Autodesk Inventor part; units mm, degrees
ref_plane "YZ Plane" through (0, 0, 0) normal (1, 0, 0) x (0, 1, 0)
ref_plane "XZ Plane" through (0, 0, 0) normal (0, 1, 0) x (-1, 0, 0)
ref_plane "XY Plane" through (0, 0, 0) normal (0, 0, 1) x (1, 0, 0)
sketch "Boceto1" plane through (0, 0, 0) normal (0, 1, 0) x (-1, 0, 0)
  line L0 (8, 8.175) -> (-8, 8.175)
  line L1 (-8, 8.175) -> (-8, -8.175)
  line L2 (-8, -8.175) -> (8, -8.175)
  line L3 (8, -8.175) -> (8, 8.175)
  point P0 (0, 0)
  dimension "d0" = 16.35
  dimension "d1" = 16
  dimension "d2" = 8
  dimension "d3" = 8.175
extrude "Extrusión1" add sketch "Boceto1" along normal mid plane 6.5
sketch "Boceto2" plane through (8, -3.25, -8.175) normal (1, 0, 0) x (0, 0, -1)
  line L0 (0, 0) -> (0, 6.5)
  line L1 (-16.35, 6.5) -> (0, 6.5)
  line L2 (-16.35, 0) -> (-16.35, 6.5)
  line L3 (0, 0) -> (-16.35, 0)
  line L4 (0, 6.5) -> (-16.35, 6.5)
  line L5 (-16.35, 6.5) -> (-14.6179, 7.5)
  line L6 (-14.6179, 7.5) -> (-14.6179, 6.5)
  line L7 (-16.35, 6.5) -> (-14.6179, 6.5)
  point P0 (-8.175, 3.25)
  dimension "d6" = 7.5
  dimension "d7" = 60
extrude "Extrusión2" add sketch "Boceto2" against normal blind 16 contours L1 L5 L6
sketch "Boceto3" plane through (-8, -3.25, 8.175) normal (0, 0, 1) x (1, 0, 0)
  line L0 (16, 0) -> (16, 6.5)
  line L1 (0, 6.5) -> (16, 6.5)
  line L2 (0, 0) -> (0, 6.5)
  line L3 (16, 0) -> (0, 0)
  circle A0 centre (13.94, 3.25) radius 0.9
  circle A1 centre (9.98, 3.25) radius 0.9
  circle A2 centre (6.02, 3.25) radius 0.9
  circle A3 centre (2.06, 3.25) radius 0.9
  point P0 (8, 3.25)
  dimension "d10" = 3.25
  dimension "P" = 3.96
  dimension "d12" = 3.96
  dimension "d13" = 3.96
  dimension "d14" = 2.06
  dimension "d15" = 1.8
  dimension "d16" = 1.8
  dimension "d17" = 1.8
  dimension "d18" = 1.8
extrude "Extrusión3" add sketch "Boceto3" along normal blind 3 contours A0 | A1 | A2 | A3
sketch "Boceto4" plane through (-8, -3.25, 8.175) normal (0, 0, 1) x (1, 0, 0)
  circle A0 centre (6.02, 3.25) radius 0.9
  circle A1 centre (9.98, 3.25) radius 0.9
  circle A2 centre (2.06, 3.25) radius 0.9
  circle A3 centre (13.94, 3.25) radius 0.9
  line L0 (16, 0) -> (16, 6.5)
  line L1 (0, 6.5) -> (16, 6.5)
  line L2 (0, 0) -> (0, 6.5)
  line L3 (16, 0) -> (0, 0)
  line L4 (8, 0) -> (16.3652, 0)
  line L5 (16.3652, 0) -> (16.3652, 8.0001)
  line L6 (16.3652, 8.0001) -> (8, 8.0001)
  line L7 (8, 8.0001) -> (8, 0)
  point P0 (8, 3.25)
extrude "Extrusión4" cut sketch "Boceto4" against normal mid plane 40 contours A1 | A3 | L3 L7 L1 L0 | L0 L1 L7 L6 L5 L4
properties part number "conector_4pines"
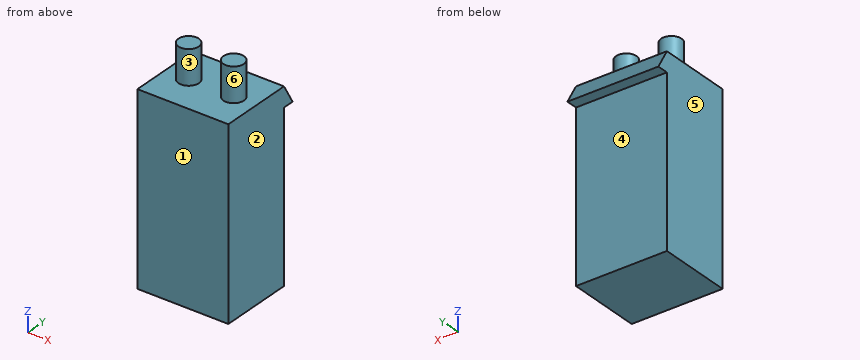
Here's how the part is built. I have some questions about the finished solid (model axes, mm). Face numbers are marked on the shaded views. A direction names the side the tool comes from. Coordinates: 2 decimals unless noted, no trailing zeros. Loops run counter-clockwise (first coordinate to the right, second up) from the corner with the lowest first, then second, coordinate; pieces in that order, holes last. Notation, with made-up numbers: (11, 86) -> (38, 86) arc R30 ccw to (38, 118) -> close; hole circle Ø6 at (21, 71). An arc over 180 degrees is marked (long way). Return JSON: item names as keys, results as strings.
1) If we section it at D-D, the plane x = -4.25: Write out the boundary of the cut face in (y, z) (3 decimals), then the cut area to 3 significant figures.
Results below:
{"outline": "(-3.25, -8.175) -> (3.25, -8.175) -> (3.25, 6.443) -> (4.25, 6.443) -> (3.25, 8.175) -> (-3.25, 8.175) -> close", "area": "107 mm²"}
2) I need wall thicknesses on line 1 (Z direction, x = -4.5, y = -1.5) (3 decimals); line 2 (Y direction, x = -4.5, z = 0); line 3 (Z direction, x = -2, y = 3.75). Which ranges of each line are inside material? Lowest first, please. Write a range as from..to.
Results below:
{"line 1": "-8.175..8.175", "line 2": "-3.25..3.25", "line 3": "6.44..7.31"}
3) For the marked faces 4, 5 and 6, which set-ups out of +Z, -Z, +X, -X, +Y, -Y let a thin tool reach every point of the face, with its end or its side?
Results below:
{"face 4": "-Z, +X, -X, +Y", "face 5": "+Z, -Z, -X, +Y, -Y", "face 6": "+Z"}
4) Will these pins go through, and if not, where does the flat tip stop? pin 1 (1.5 mm diameter, centred on y = 0.5, z = 9, fed in from +X); pin 2 (2.5 mm diameter, centred on x = -3.5, z = -3.5, fed in from +Y).
Results below:
{"pin 1": "x = -1.08", "pin 2": "y = 3.25"}
5) If we section it at C-C, the plane z = -2: Write out the boundary of the cut face in (x, y).
Results below:
{"outline": "(-8, -3.25) -> (0, -3.25) -> (0, 3.25) -> (-8, 3.25) -> close"}
6) Thinking about a two-plate mould opening in X: for the marked faces 1, 2 and 3, which applies, +X half, -X half, draft (parallel to the pull), parting line (faces both ways), or undercut?
Results below:
{"face 1": "draft", "face 2": "+X half", "face 3": "undercut"}
7) If we section it at B-B, the plane y = -0.5: Write out the boundary of the cut face in (x, z) (3 decimals).
Results below:
{"outline": "(-8, -8.175) -> (0, -8.175) -> (0, 8.175) -> (-1.232, 8.175) -> (-1.232, 11.175) -> (-2.728, 11.175) -> (-2.728, 8.175) -> (-5.192, 8.175) -> (-5.192, 11.175) -> (-6.688, 11.175) -> (-6.688, 8.175) -> (-8, 8.175) -> close"}
8) If we section it at A-A, the plane x = -1.98: Write out the boundary of the cut face in (y, z) (3 decimals).
Results below:
{"outline": "(-3.25, -8.175) -> (3.25, -8.175) -> (3.25, 6.443) -> (4.25, 6.443) -> (3.25, 8.175) -> (0.9, 8.175) -> (0.9, 11.175) -> (-0.9, 11.175) -> (-0.9, 8.175) -> (-3.25, 8.175) -> close"}
